```python
from build123d import *

# Parameters (mm, degrees)
F1_DEPTH = 4.7625
F2_R     = 9.525
F3_DEPTH = 4.7635
F4_SIZE  = 1.5875


# Not quite as in the source:
# - a feature of the source that left no trace in its solid (it failed there, or was rolled back) is left out


with BuildPart() as f1:
    # F0 (on Top) → F1 (new body)
    with BuildSketch(Plane.XY):
        Polygon((-3.074264621, 21.805118867), (-40.0660246394, 41.4531760826), (-21.6879004002, 3.8143528936), (-51.8053957451, -25.295317935), (-10.3295949709, -19.4477191337), (8.0485292683, -57.0865423226), (15.3038596181, -15.8337043219), (56.7796603923, -9.9861055206), (19.787900374, 9.6619516949), (27.0432307238, 50.9147896956), align=None)
    extrude(amount=F1_DEPTH)

    # F2 (on Top) → F3 (cut, through all)
    with BuildSketch(Plane.XY):
        with Locations((15.3038596181, -15.8337043219)):
            Circle(F2_R)
        with Locations((-10.3295949709, -19.4477191337)):
            Circle(F2_R)
        with Locations((-21.6879004002, 3.8143528936)):
            Circle(F2_R)
        with Locations((-3.074264621, 21.805118867)):
            Circle(F2_R)
        with Locations((19.787900374, 9.6619516949)):
            Circle(F2_R)
    extrude(amount=F3_DEPTH, mode=Mode.SUBTRACT)

    # F4
    f4_edges = [f1.edges().sort_by_distance(p)[0] for p in [
        (24.240507, 34.97888, 4.7625),
        (15.408887, 39.669767, 4.7625),
        (-1.744503, 12.373398, 4.7625),
        (-25.776163, 33.863161, 4.7625),
        (-32.966583, 26.913355, 4.7625),
        (-12.306882, 2.164469, 4.7625),
        (-40.171052, -14.050296, 4.7625),
        (-35.783356, -23.036399, 4.7625),
        (-5.861568, -11.035682, 4.7625),
        (0.949087, -42.546721, 4.7625),
        (10.851253, -41.150633, 4.7625),
        (8.684234, -8.984896, 4.7625),
        (40.75762, -12.245024, 4.7625),
        (42.489799, -2.39609, 4.7625),
        (11.22872, 5.482711, 4.7625),
        (24.240507, 34.97888, 0),
        (15.408887, 39.669767, 0),
        (-1.744503, 12.373398, 0),
        (-25.776163, 33.863161, 0),
        (-32.966583, 26.913355, 0),
        (-12.306882, 2.164469, 0),
        (-40.171052, -14.050296, 0),
        (-35.783356, -23.036399, 0),
        (-5.861568, -11.035682, 0),
        (0.949087, -42.546721, 0),
        (10.851253, -41.150633, 0),
        (8.684234, -8.984896, 0),
        (40.75762, -12.245024, 0),
        (42.489799, -2.39609, 0),
        (11.22872, 5.482711, 0),
    ]]
    chamfer(f4_edges, length=F4_SIZE)


solid = f1.part
```
Geometry check sheet. Reference: the model listing, model coordinates, mm. A direction names the side the tool comes from. Give positions to 0.01 mm unless a question says otherwise; leave off trailing zeros. Loops run counter-clockwise (first coordinate to the right, second up) from the corner with the lowest first, then second, coordinate; pieces in that order, holes last. Notation, with made-up numbers: M -21.75,81.25 L -4.75,81.25 A23 cw -4.75,95.25 Z; hole C -38,80 d6. An arc over 180 degrees is marked long. Write item = value, one per line. Start each with the question number.
1. Go/stop test with flat-tipped pins: P1, Ø22, axis at x = 15.3, y = -15.83, coming from the +Z side; P2, Ø22, axis at x = -10.33, y = -19.45, coming from the -Z side; P3, Ø2, axis at x = 15, z = 1, coming from the +Y side. Record where each tip stops, or that it passes through.
2. Tool access check on faces 1 (the face through (24.2, 34.76, 2.37)), 2 (the face through (23.41, 34.9, 3.98)), 3 (the face through (-36.12, -22.27, 0.78)). Record the directions out of +Z, -Z, +X, -X, +Y, -Y that give a thin tool (end or side, any length) a straight path to the whole face; none if there is none.
3. Section check A-A, the plane z = 2.4. Enter the section's corners in (x, y) (3 decimals), plus the area to 3 significant figures.
4. Section check B-B, the plane y = 34. Enter the section's corners in (x, z) (1 decimal), plus the area to 3 significant figures.
5. Section check D-D, the plane x = -34. Enter the section's corners in (y, z) (1 decimal).
6. Draft check along Y on faces 4 (the face through (2, 1, 0)), 5 (the face through (-32.36, 27.46, 3.96)), 6 (the face through (1.6, -42, 4)). Enter one of: +Y half, -Y half, draft (parallel to the pull), parting line (faces both ways), or undercut.
7. Section check C-C, the plane x = 42.5. Enter the section's corners in (y, z) (1 decimal).
8. Thickness scan on probe 1 along Y at (x, z) = (16, 0.35); probe 2 along Y at (x, z) = (14, 1.35); probe 3 along X at (y, z) = (13, 3.85). Record the ranges inside material, lowest first.
Values follow:
q1.P1 = 4.66
q1.P2 = 0.11
q1.P3 = 40.06
q2.face_1 = +Z, -Z, +X
q2.face_2 = +Z, +X
q2.face_3 = -Z, -Y
q3.outline = M -51.805,-25.295 L -19.761,-20.777 A9.525 cw long -6.15,-28.007 L 8.049,-57.087 L 13.654,-25.215 A9.525 cw long 24.736,-14.504 L 56.78,-9.986 L 28.2,5.194 A9.525 cw long 21.438,19.043 L 27.043,50.915 L 3.775,28.425 A9.525 cw long -11.486,26.273 L -40.066,41.453 L -25.867,12.374 A9.525 cw long -28.537,-2.805 Z
q3.area = 2,730 mm^2
q4.outline = M -36.4,1.6 L -34.7,0 L -29.4,0 L -26,1.6 L -26,3.2 L -29.4,4.8 L -34.7,4.8 L -36.4,3.2 Z; M 9.5,1.6 L 11.8,0 L 22.5,0 L 24.1,1.6 L 24.1,3.2 L 22.5,4.8 L 11.8,4.8 L 9.5,3.2 Z
q4.area = 104 mm^2
q5.outline = M -22.8,1.6 L -21.2,0 L -10.3,0 L -8.1,1.6 L -8.1,3.2 L -10.3,4.8 L -21.2,4.8 L -22.8,3.2 Z; M 29,1.6 L 32.6,0 L 36.4,0 L 38.2,1.6 L 38.2,3.2 L 36.4,4.8 L 32.6,4.8 L 29,3.2 Z
q6.face_4 = draft
q6.face_5 = undercut
q6.face_6 = -Y half
q7.outline = M -12,1.6 L -10.4,0 L -4.2,0 L -2.4,1.6 L -2.4,3.2 L -4.2,4.8 L -10.4,4.8 L -12,3.2 Z
q8.probe_1 = -5.09 to -0.41, 19.74 to 38.52
q8.probe_2 = -6.16 to 1.8, 17.52 to 37.98
q8.probe_3 = -17.25 to -8.22, 2.07 to 10.15
